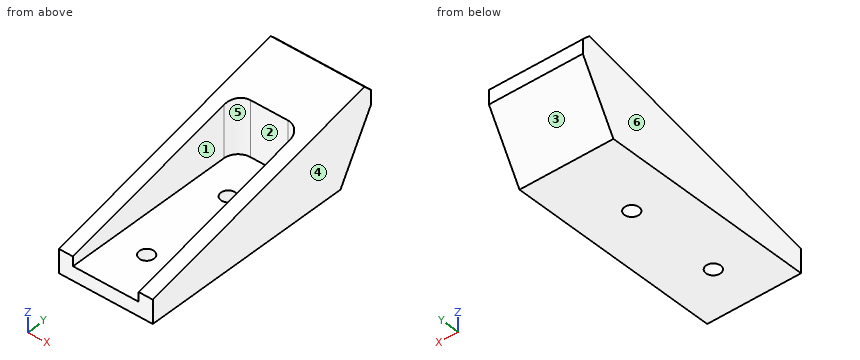
from build123d import *

# Parameters (mm, degrees)
BOSS_EXTRUDE1_DEPTH = 20
CUT_EXTRUDE1_START  = -14.990381
SKETCH4_W           = 14
SKETCH4_H           = 40
CUT_EXTRUDE1_DEPTH  = 11.712434
FILLET1_R           = 3
CHAMFER1_SIZE2      = 2
CHAMFER1_SIZE       = 1.656014526
M3_CLEARANCE_D      = 3.099999896


with BuildPart() as part:
    # Sketch1 → Boss-Extrude1 (new body)
    with BuildSketch(Plane(origin=(0, 0, 0), x_dir=(0, 0, -1), z_dir=(1, 0, 0))):
        Polygon((0, 0), (-5, 0), (-17.990381057, 53.5), (-12.990381057, 53.5), (0, 46), align=None)
    extrude(amount=BOSS_EXTRUDE1_DEPTH)

    # Sketch4 → Cut-Extrude1 (cut)
    with BuildSketch(Plane.XY.offset(17.990381057).offset(CUT_EXTRUDE1_START)):
        with Locations((10, 20)):
            Rectangle(SKETCH4_W, SKETCH4_H)
    extrude(amount=CUT_EXTRUDE1_DEPTH, mode=Mode.SUBTRACT)

    # Fillet1
    fillet1_edges = [part.edges().sort_by_distance(p)[0] for p in [
        (3, 40, 8.856217057),
        (17, 40, 8.856217057),
    ]]
    fillet(fillet1_edges, radius=FILLET1_R)

    # Chamfer1
    chamfer1_edges = [part.edges().sort_by_distance(p)[0] for p in [
        (10, 53.5, 17.990381057),
    ]]
    chamfer(chamfer1_edges, length=CHAMFER1_SIZE, length2=CHAMFER1_SIZE2)

    # M3 Clearance (through all)
    with Locations(Plane(origin=(10, 30, 3), x_dir=(1, 0, 0), z_dir=(0, 0, 1))):
        with Locations((0, 0), (0, -20)):
            Hole(M3_CLEARANCE_D / 2)


solid = part.part
Model file for the job. Use its own axes, mm. Face numbers are marked on the shaded views. A direction names the side the tool comes from. Give positions to 0.01 mm unless a question says otherwise; leave off trailing zeros. Write each loop counter-clockwise with the first axis right and the second up, starting at its lowest first coordinate (ties: lowest second). Pieces come first, ordered by that corner, then holes. Notation, with made-up numbers: (85.5, 54) -> (124.5, 54) arc R19 ccw to (124.5, 78) -> close; hole circle Ø3 at (59.25, 0). An arc over 180 degrees is marked (long way). Write item = value, one per line.
(1) Slice it at C-C, the plane x = 7.5. Give the cut face in (y, z), then the cut area to 3 significant figures.
Determined:
outline = (0, 0) -> (46, 0) -> (53.5, 12.99) -> (53.5, 15.99) -> (51.89, 17.6) -> (40, 14.71) -> (40, 3) -> (0, 3) -> close
area = 290 mm2
(2) Mould opens along X. For the marked faces 1, 2, 3 and 4 say: released by +X, released by -X, zero draft, split by the parting line, or undercut.
Determined:
face_1 = undercut
face_2 = undercut
face_3 = zero draft
face_4 = released by +X
(3) Slice it at A-A, the plane x = 10. Give the cut face in (y, z).
Determined:
outline = (0, 0) -> (8.45, 0) -> (8.45, 3) -> (0, 3) -> close; (11.55, 0) -> (28.45, 0) -> (28.45, 3) -> (11.55, 3) -> close; (31.55, 0) -> (46, 0) -> (53.5, 12.99) -> (53.5, 15.99) -> (51.89, 17.6) -> (40, 14.71) -> (40, 3) -> (31.55, 3) -> close
(4) Slice it at B-B, the plane y = 11. Give the cut face in (x, z), then the cut area to 3 significant figures.
Determined:
outline = (0, 0) -> (8.82, 0) -> (8.82, 3) -> (3, 3) -> (3, 7.67) -> (0, 7.67) -> close; (11.18, 0) -> (20, 0) -> (20, 7.67) -> (17, 7.67) -> (17, 3) -> (11.18, 3) -> close
area = 80.9 mm2
(5) Slice it at D-D, the plane y = 24. Give the cut face in (x, z).
Determined:
outline = (0, 0) -> (20, 0) -> (20, 10.83) -> (17, 10.83) -> (17, 3) -> (3, 3) -> (3, 10.83) -> (0, 10.83) -> close
(6) Tool access for the marked faces 5 and 6: list every direction of +Z, -Z, +X, -X, +Y, -Y with a clear straight run to the whole face (end or side of a thin tool).
Determined:
face_5 = +Z, -Y
face_6 = +Z, -Z, -X, +Y, -Y
(7) Flat gauge pins, fed straight in: P1, Ø1.5, axis at x = 13, z = 7.5, coming from the -Y side; P2, Ø4, axis at x = 10.5, y = 18.5, coming from the +Z side; P3, Ø10, axis at x = 16, y = 33, coming from the +Z side. Where does each tip first touch, or does it go through?
Determined:
P1 = 40
P2 = 3
P3 = 14.21
(8) Probe line 1 along Y through (x, z) = (10, 2.4); line 2 along X through (y, z) = (36.5, 13); line 3 along Y through (x, z) = (10, 1.55). List the from-to ranges inside material, lowest first.
Determined:
line_1 = 0 to 8.45, 11.55 to 28.45, 31.55 to 47.39
line_2 = 0 to 3, 17 to 20
line_3 = 0 to 8.45, 11.55 to 28.45, 31.55 to 46.89
